Build history of the part. All positions in model axes, mm. A direction names the side the tool comes from. Give positions to 0.01 mm unless a question says otherwise; leave off trailing zeros. Order: outer loops, then holes, each group sorted by start corner. A loop starts at its lowest first (then second) coordinate and runs counter-clockwise, first axis right, second up. Notation, with made-up numbers: M 60.25,65 L 73.25,65 A27 ccw 73.25,82 Z; hole C 35,40 d2. An arc over 180 degrees is marked long. One line per item, written item: value.
from build123d import *

# Parameters (mm, degrees)
SKETCH_1_W          = 230
SKETCH_1_H          = 150
EXTRUDE_1_DEPTH     = 42
CUT_EXTRUDE_2_DEPTH = 40
FILLET_1_R          = 5
FILLET_2_R          = 5
SKETCH_5_R          = 2.5
CUT_EXTRUDE_3_DEPTH = 43
SKETCH_6_R          = 12.5
CUT_EXTRUDE_4_DEPTH = 10
CUT_EXTRUDE_5_REACH = 232
SKETCH_9_R          = 2
SKETCH_9_R_2        = 1


with BuildPart() as part:
    # 草图1 → 凸台-拉伸1 (new body)
    with BuildSketch(Plane(origin=(0, 0, 0), x_dir=(1, 0, 0), z_dir=(0, 1, 0))):
        with Locations((115, 75)):
            Rectangle(SKETCH_1_W, SKETCH_1_H)
    extrude(amount=EXTRUDE_1_DEPTH)

    # 草图4 → 切除-拉伸2 (cut)
    with BuildSketch(Plane(origin=(0, 42, 0), x_dir=(1, 0, 0), z_dir=(0, 1, 0))):
        Polygon((2, 125.5), (2, 24.5), (15.5, 24.5), (15.5, 2), (214.5, 2), (214.5, 24.5), (228, 24.5), (228, 125.5), (214.5, 125.5), (214.5, 148), (15.5, 148), (15.5, 125.5), align=None)
    extrude(amount=-CUT_EXTRUDE_2_DEPTH, mode=Mode.SUBTRACT)

    # 圆角1
    fillet_1_edges = [part.edges().sort_by_distance(p)[0] for p in [
        (0, 21, -150),
        (0, 21, 0),
        (230, 21, 0),
        (230, 21, -150),
    ]]
    fillet(fillet_1_edges, radius=FILLET_1_R)

    # 圆角2
    fillet_2_edges = [part.edges().sort_by_distance(p)[0] for p in [
        (2, 22, -125.5),
        (15.5, 22, -125.5),
        (15.5, 22, -148),
        (214.5, 22, -148),
        (214.5, 22, -125.5),
        (228, 22, -125.5),
        (228, 22, -24.5),
        (214.5, 22, -24.5),
        (214.5, 22, -2),
        (15.5, 22, -2),
        (15.5, 22, -24.5),
        (2, 22, -24.5),
    ]]
    fillet(fillet_2_edges, radius=FILLET_2_R)

    # 草图5 → 切除-拉伸3 (cut, through all)
    with BuildSketch(Plane(origin=(0, 42, 0), x_dir=(1, 0, 0), z_dir=(0, 1, 0))):
        with Locations((222, 142)):
            Circle(SKETCH_5_R)
        with Locations((6.63178387, 8)):
            Circle(SKETCH_5_R)
        with Locations((222, 8)):
            Circle(SKETCH_5_R)
        with Locations((8, 142)):
            Circle(SKETCH_5_R)
    extrude(amount=-CUT_EXTRUDE_3_DEPTH, mode=Mode.SUBTRACT)

    # 草图6 → 切除-拉伸4 (cut)
    with BuildSketch(Plane(origin=(230, 0, 0), x_dir=(0, 0, -1), z_dir=(1, 0, 0))):
        with Locations((50, 21)):
            Circle(SKETCH_6_R)
    extrude(amount=-CUT_EXTRUDE_4_DEPTH, mode=Mode.SUBTRACT)

    # 草图9 → 切除-拉伸5 (cut, up to next)
    with BuildSketch(Plane(origin=(230, 0, 0), x_dir=(0, 0, -1), z_dir=(1, 0, 0)), mode=Mode.PRIVATE) as cut_extrude_5_sk1:
        with Locations((100, 21)):
            Circle(SKETCH_9_R)
    cut_extrude_5_tool1 = extrude(cut_extrude_5_sk1.sketch, amount=-CUT_EXTRUDE_5_REACH, mode=Mode.PRIVATE) & part.part
    add(cut_extrude_5_tool1.solids().sort_by_distance((230, 21, -100))[0], mode=Mode.SUBTRACT)
    # 草图9 → 切除-拉伸5 (cut, up to next)
    with BuildSketch(Plane(origin=(230, 0, 0), x_dir=(0, 0, -1), z_dir=(1, 0, 0)), mode=Mode.PRIVATE) as cut_extrude_5_sk2:
        with Locations((103.04364251, 24.966893025)):
            Circle(SKETCH_9_R_2)
    cut_extrude_5_tool2 = extrude(cut_extrude_5_sk2.sketch, amount=-CUT_EXTRUDE_5_REACH, mode=Mode.PRIVATE) & part.part
    add(cut_extrude_5_tool2.solids().sort_by_distance((230, 24.966893, -103.043643))[0], mode=Mode.SUBTRACT)
    # 草图9 → 切除-拉伸5 (cut, up to next)
    with BuildSketch(Plane(origin=(230, 0, 0), x_dir=(0, 0, -1), z_dir=(1, 0, 0)), mode=Mode.PRIVATE) as cut_extrude_5_sk3:
        with Locations((104.869828016, 27.34702884)):
            Circle(SKETCH_9_R_2)
    cut_extrude_5_tool3 = extrude(cut_extrude_5_sk3.sketch, amount=-CUT_EXTRUDE_5_REACH, mode=Mode.PRIVATE) & part.part
    add(cut_extrude_5_tool3.solids().sort_by_distance((230, 27.347029, -104.869828))[0], mode=Mode.SUBTRACT)
    # 草图9 → 切除-拉伸5 (cut, up to next)
    with BuildSketch(Plane(origin=(230, 0, 0), x_dir=(0, 0, -1), z_dir=(1, 0, 0)), mode=Mode.PRIVATE) as cut_extrude_5_sk4:
        with Locations((104.957197217, 21.6528367)):
            Circle(SKETCH_9_R_2)
    cut_extrude_5_tool4 = extrude(cut_extrude_5_sk4.sketch, amount=-CUT_EXTRUDE_5_REACH, mode=Mode.PRIVATE) & part.part
    add(cut_extrude_5_tool4.solids().sort_by_distance((230, 21.652837, -104.957197))[0], mode=Mode.SUBTRACT)
    # 草图9 → 切除-拉伸5 (cut, up to next)
    with BuildSketch(Plane(origin=(230, 0, 0), x_dir=(0, 0, -1), z_dir=(1, 0, 0)), mode=Mode.PRIVATE) as cut_extrude_5_sk5:
        with Locations((103.966893025, 17.95635749)):
            Circle(SKETCH_9_R_2)
    cut_extrude_5_tool5 = extrude(cut_extrude_5_sk5.sketch, amount=-CUT_EXTRUDE_5_REACH, mode=Mode.PRIVATE) & part.part
    add(cut_extrude_5_tool5.solids().sort_by_distance((230, 17.956357, -103.966893))[0], mode=Mode.SUBTRACT)
    # 草图9 → 切除-拉伸5 (cut, up to next)
    with BuildSketch(Plane(origin=(230, 0, 0), x_dir=(0, 0, -1), z_dir=(1, 0, 0)), mode=Mode.PRIVATE) as cut_extrude_5_sk6:
        with Locations((100.6528367, 16.042802783)):
            Circle(SKETCH_9_R_2)
    cut_extrude_5_tool6 = extrude(cut_extrude_5_sk6.sketch, amount=-CUT_EXTRUDE_5_REACH, mode=Mode.PRIVATE) & part.part
    add(cut_extrude_5_tool6.solids().sort_by_distance((230, 16.042803, -100.652837))[0], mode=Mode.SUBTRACT)
    # 草图9 → 切除-拉伸5 (cut, up to next)
    with BuildSketch(Plane(origin=(230, 0, 0), x_dir=(0, 0, -1), z_dir=(1, 0, 0)), mode=Mode.PRIVATE) as cut_extrude_5_sk7:
        with Locations((96.95635749, 17.033106975)):
            Circle(SKETCH_9_R_2)
    cut_extrude_5_tool7 = extrude(cut_extrude_5_sk7.sketch, amount=-CUT_EXTRUDE_5_REACH, mode=Mode.PRIVATE) & part.part
    add(cut_extrude_5_tool7.solids().sort_by_distance((230, 17.033107, -96.956357))[0], mode=Mode.SUBTRACT)
    # 草图9 → 切除-拉伸5 (cut, up to next)
    with BuildSketch(Plane(origin=(230, 0, 0), x_dir=(0, 0, -1), z_dir=(1, 0, 0)), mode=Mode.PRIVATE) as cut_extrude_5_sk8:
        with Locations((95.042802783, 20.3471633)):
            Circle(SKETCH_9_R_2)
    cut_extrude_5_tool8 = extrude(cut_extrude_5_sk8.sketch, amount=-CUT_EXTRUDE_5_REACH, mode=Mode.PRIVATE) & part.part
    add(cut_extrude_5_tool8.solids().sort_by_distance((230, 20.347163, -95.042803))[0], mode=Mode.SUBTRACT)
    # 草图9 → 切除-拉伸5 (cut, up to next)
    with BuildSketch(Plane(origin=(230, 0, 0), x_dir=(0, 0, -1), z_dir=(1, 0, 0)), mode=Mode.PRIVATE) as cut_extrude_5_sk9:
        with Locations((96.033106975, 24.04364251)):
            Circle(SKETCH_9_R_2)
    cut_extrude_5_tool9 = extrude(cut_extrude_5_sk9.sketch, amount=-CUT_EXTRUDE_5_REACH, mode=Mode.PRIVATE) & part.part
    add(cut_extrude_5_tool9.solids().sort_by_distance((230, 24.043643, -96.033107))[0], mode=Mode.SUBTRACT)
    # 草图9 → 切除-拉伸5 (cut, up to next)
    with BuildSketch(Plane(origin=(230, 0, 0), x_dir=(0, 0, -1), z_dir=(1, 0, 0)), mode=Mode.PRIVATE) as cut_extrude_5_sk10:
        with Locations((99.3471633, 25.957197217)):
            Circle(SKETCH_9_R_2)
    cut_extrude_5_tool10 = extrude(cut_extrude_5_sk10.sketch, amount=-CUT_EXTRUDE_5_REACH, mode=Mode.PRIVATE) & part.part
    add(cut_extrude_5_tool10.solids().sort_by_distance((230, 25.957197, -99.347163))[0], mode=Mode.SUBTRACT)
    # 草图9 → 切除-拉伸5 (cut, up to next)
    with BuildSketch(Plane(origin=(230, 0, 0), x_dir=(0, 0, -1), z_dir=(1, 0, 0)), mode=Mode.PRIVATE) as cut_extrude_5_sk11:
        with Locations((107.931515546, 22.04453872)):
            Circle(SKETCH_9_R_2)
    cut_extrude_5_tool11 = extrude(cut_extrude_5_sk11.sketch, amount=-CUT_EXTRUDE_5_REACH, mode=Mode.PRIVATE) & part.part
    add(cut_extrude_5_tool11.solids().sort_by_distance((230, 22.044539, -107.931516))[0], mode=Mode.SUBTRACT)
    # 草图9 → 切除-拉伸5 (cut, up to next)
    with BuildSketch(Plane(origin=(230, 0, 0), x_dir=(0, 0, -1), z_dir=(1, 0, 0)), mode=Mode.PRIVATE) as cut_extrude_5_sk12:
        with Locations((106.34702884, 16.130171984)):
            Circle(SKETCH_9_R_2)
    cut_extrude_5_tool12 = extrude(cut_extrude_5_sk12.sketch, amount=-CUT_EXTRUDE_5_REACH, mode=Mode.PRIVATE) & part.part
    add(cut_extrude_5_tool12.solids().sort_by_distance((230, 16.130172, -106.347029))[0], mode=Mode.SUBTRACT)
    # 草图9 → 切除-拉伸5 (cut, up to next)
    with BuildSketch(Plane(origin=(230, 0, 0), x_dir=(0, 0, -1), z_dir=(1, 0, 0)), mode=Mode.PRIVATE) as cut_extrude_5_sk13:
        with Locations((101.04453872, 13.068484454)):
            Circle(SKETCH_9_R_2)
    cut_extrude_5_tool13 = extrude(cut_extrude_5_sk13.sketch, amount=-CUT_EXTRUDE_5_REACH, mode=Mode.PRIVATE) & part.part
    add(cut_extrude_5_tool13.solids().sort_by_distance((230, 13.068484, -101.044539))[0], mode=Mode.SUBTRACT)
    # 草图9 → 切除-拉伸5 (cut, up to next)
    with BuildSketch(Plane(origin=(230, 0, 0), x_dir=(0, 0, -1), z_dir=(1, 0, 0)), mode=Mode.PRIVATE) as cut_extrude_5_sk14:
        with Locations((95.130171984, 14.65297116)):
            Circle(SKETCH_9_R_2)
    cut_extrude_5_tool14 = extrude(cut_extrude_5_sk14.sketch, amount=-CUT_EXTRUDE_5_REACH, mode=Mode.PRIVATE) & part.part
    add(cut_extrude_5_tool14.solids().sort_by_distance((230, 14.652971, -95.130172))[0], mode=Mode.SUBTRACT)
    # 草图9 → 切除-拉伸5 (cut, up to next)
    with BuildSketch(Plane(origin=(230, 0, 0), x_dir=(0, 0, -1), z_dir=(1, 0, 0)), mode=Mode.PRIVATE) as cut_extrude_5_sk15:
        with Locations((92.068484454, 19.95546128)):
            Circle(SKETCH_9_R_2)
    cut_extrude_5_tool15 = extrude(cut_extrude_5_sk15.sketch, amount=-CUT_EXTRUDE_5_REACH, mode=Mode.PRIVATE) & part.part
    add(cut_extrude_5_tool15.solids().sort_by_distance((230, 19.955461, -92.068484))[0], mode=Mode.SUBTRACT)
    # 草图9 → 切除-拉伸5 (cut, up to next)
    with BuildSketch(Plane(origin=(230, 0, 0), x_dir=(0, 0, -1), z_dir=(1, 0, 0)), mode=Mode.PRIVATE) as cut_extrude_5_sk16:
        with Locations((93.65297116, 25.869828016)):
            Circle(SKETCH_9_R_2)
    cut_extrude_5_tool16 = extrude(cut_extrude_5_sk16.sketch, amount=-CUT_EXTRUDE_5_REACH, mode=Mode.PRIVATE) & part.part
    add(cut_extrude_5_tool16.solids().sort_by_distance((230, 25.869828, -93.652971))[0], mode=Mode.SUBTRACT)
    # 草图9 → 切除-拉伸5 (cut, up to next)
    with BuildSketch(Plane(origin=(230, 0, 0), x_dir=(0, 0, -1), z_dir=(1, 0, 0)), mode=Mode.PRIVATE) as cut_extrude_5_sk17:
        with Locations((98.95546128, 28.931515546)):
            Circle(SKETCH_9_R_2)
    cut_extrude_5_tool17 = extrude(cut_extrude_5_sk17.sketch, amount=-CUT_EXTRUDE_5_REACH, mode=Mode.PRIVATE) & part.part
    add(cut_extrude_5_tool17.solids().sort_by_distance((230, 28.931516, -98.955461))[0], mode=Mode.SUBTRACT)


solid = part.part
1) Saw through at C-C, the plane y = 39. Give the number of separate pieces and of enclosed holes in the cut face, then the cut area to 3 significant figures.
Check values:
separate pieces: 1
enclosed holes: 5
area: 2,640 mm^2
2) Tool access for faces 1 (the face through (116, 22, -148)), 2 (the face through (228, 21, -1)): list every direction of +Z, -Z, +X, -X, +Y, -Y with a clear straight run to the whole face (end or side of a thin tool).
Check values:
face 1: +Y
face 2: +Z, +X, +Y, -Y
3) Pin check, flat tips, straight feed: pin 1 (3 mm diameter, centred on x = 222, z = -142, fed in from -Y); pin 2 (1.8 mm diameter, centred on y = 17.03, z = -96.96, fed in from +X); pin 3 (2.5 mm diameter, centred on y = 24.04, z = -96.03, fed in from +X); pin 4 (1 mm diameter, centred on x = 24, z = -59, fed in from +Y). Stop position of each tip, or through.
Check values:
pin 1: through
pin 2: x = 2
pin 3: x = 230
pin 4: y = 2
4) Mould opens along X. For faces 3 (the face through (7.67, 21.29, -144.48)), 4 (the face through (3.43, 21.72, -26)), 5 (the face through (228, 21, -149)), 6 (the face through (113, 21, -150)) say: released by +X, released by -X, zero draft, split by the parting line, or undercut.
Check values:
face 3: undercut
face 4: undercut
face 5: released by +X
face 6: zero draft
5) Saw through at A-A, the plane z = -50. Write the cut outline in (x, y).
Check values:
outline: M 0,0 L 230,0 L 230,8.5 L 228,8.5 L 228,2 L 2,2 L 2,42 L 0,42 Z; M 228,33.5 L 230,33.5 L 230,42 L 228,42 Z
6) Drill centre lines: probe 1 along X at (y, z) = (38, -7.5); probe 2 along Z at (x, y) = (222, 28.5); probe 3 along X at (y, z) = (21, -138). Where is each one in solid material? Low to high. Write a range as from..to.
Check values:
probe 1: 0..4.18, 9.08..15.5, 214.5..219.55, 224.45..230
probe 2: -150..-144.5, -139.5..-125.5, -24.5..-10.5, -5.5..0
probe 3: 0..15.5, 214.5..230
7) Saw through at B-B, the plane x = 104.5. Write the cut outline in (y, z).
Check values:
outline: M 0,-150 L 42,-150 L 42,-148 L 2,-148 L 2,-2 L 42,-2 L 42,0 L 0,0 Z
